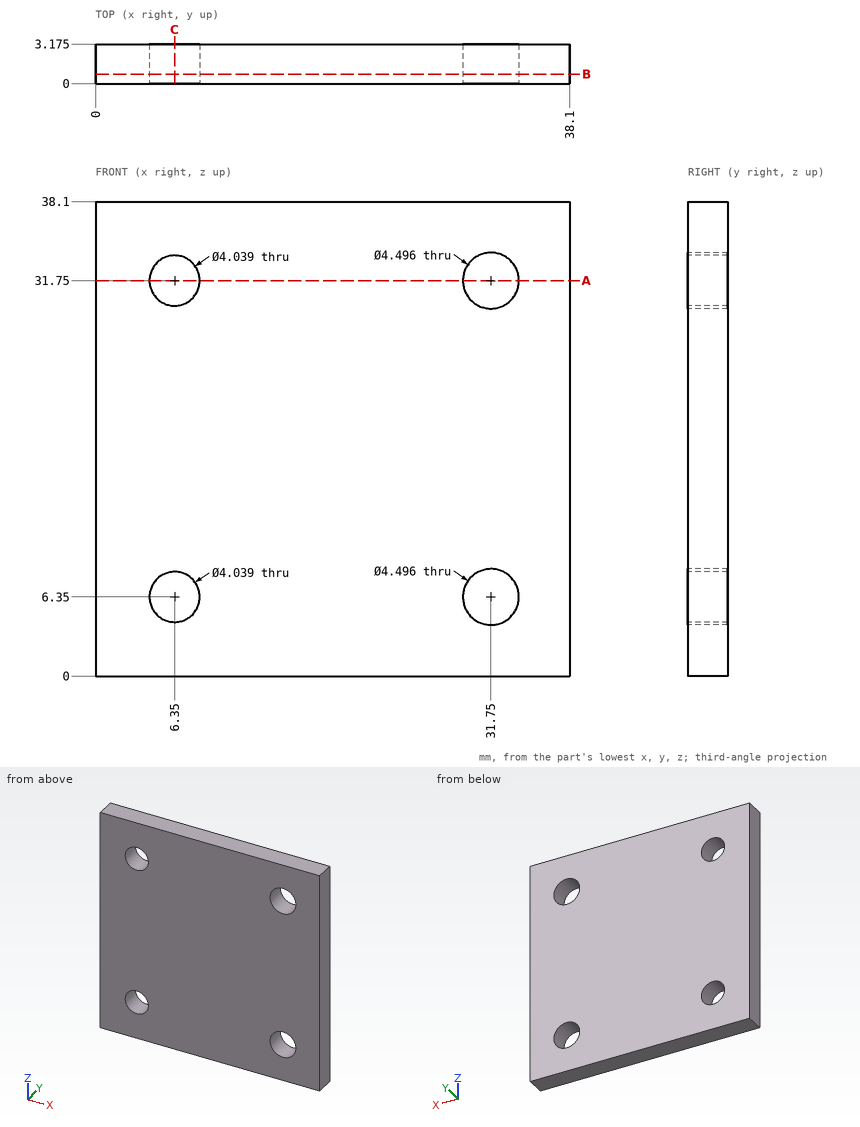
Answer from the drawing. Dimensions are ordinates in mm from the lowest x, y and z of the part. Round coordinates to 2 decimals unless told otherwise and drop trailing zeros. Write each loop counter-clockwise with the first axis right and the second up, starting at its lowest first coordinate (ties: lowest second). Pieces come first, ordered by that corner, then holes. Notation, with made-up numbers: (-25, -15.75) -> (33, -15.75) arc R17 ccw to (33, 4.25) -> close; hole circle Ø4 at (13, -30). An arc over 180 degrees is marked (long way). Answer in a Markdown table with one row per item. Add a question column.
1) Find section B-B, the plane y = 0.75. State how many separate pieces and enclosed holes the cut face has, and give its area (3 significant figures).
2) Find section C-C, the plane x = 6.35. Determine the outline of the cut face in (y, z) (1 decimal).
3) Find section A-A, the plane z = 31.75. Determine the outline of the cut face in (x, y) (1 decimal).
4) Consider line 1 (Z direction, x = 6.35, y = 2.2); line 2 (X direction, y = 2, z = 31.75); line 3 (Z direction, x = 31.75, y = 2.05). Determine where each line is inside the solid, lowest interval first.
5) Given P1, Ø1, axis at y = 2.5, z = 17.5, coming from the -X side; P2, Ø2.5, axis at x = 31.75, z = 31.75, coming from the -Y side, each flat-ended and moving along its own axis, determine where each tip first touches the part or whether it passes through.
Findings below:
| question | item | result |
|---|---|---|
| 1 | separate pieces | 1 |
| 1 | enclosed holes | 4 |
| 1 | area | 1,390 mm² |
| 2 | outline | (0, 0) -> (3.2, 0) -> (3.2, 4.3) -> (0, 4.3) -> close; (0, 8.4) -> (3.2, 8.4) -> (3.2, 29.7) -> (0, 29.7) -> close; (0, 33.8) -> (3.2, 33.8) -> (3.2, 38.1) -> (0, 38.1) -> close |
| 3 | outline | (0, 0) -> (4.3, 0) -> (4.3, 3.2) -> (0, 3.2) -> close; (8.4, 0) -> (29.5, 0) -> (29.5, 3.2) -> (8.4, 3.2) -> close; (34, 0) -> (38.1, 0) -> (38.1, 3.2) -> (34, 3.2) -> close |
| 4 | line 1 | 0 to 4.33, 8.37 to 29.73, 33.77 to 38.1 |
| 4 | line 2 | 0 to 4.33, 8.37 to 29.5, 34 to 38.1 |
| 4 | line 3 | 0 to 4.1, 8.6 to 29.5, 34 to 38.1 |
| 5 | P1 | x = 0 |
| 5 | P2 | through |
